Autodesk Inventor part; units mm, degrees
ref_plane "YZ Plane" through (0, 0, 0) normal (1, 0, 0) x (0, 1, 0)
ref_plane "XZ Plane" through (0, 0, 0) normal (0, 1, 0) x (-1, 0, 0)
ref_plane "XY Plane" through (0, 0, 0) normal (0, 0, 1) x (1, 0, 0)
sketch "Sketch1" plane through (0, 0, 0) normal (0, 0, 1) x (1, 0, 0)
  line L0 (-750, 50) -> (750, 50)
  line L1 (750, 50) -> (750, 0)
  line L2 (750, 0) -> (-750, 0)
  line L3 (-750, 0) -> (-750, 50)
  point P0 (0, 0)
  point P1 (0, 0)
  dimension "d0" = 1500
  dimension "d1" = 50
extrude "Plate1" add sketch "Sketch1" along normal blind 3
sketch "Sketch2" plane through (750, 3, 0) normal (0, -1, 0) x (1, 0, 0)
  line L0 (-1500, 0) -> (0, 0)
  line L1 (0, 0) -> (0, 30)
  line L2 (0, 30) -> (-1500, 30)
  line L3 (-1500, 30) -> (-1500, 0)
edge flange "Flange1" height 30 angle 90 thickness 3 bend radius 3 thickness toward (0, -1, 0) relief tear relief width 3 relief depth 1.5 edges at (0, 0, 3) wall of the first edge with corners at (-750, 3, 0) (750, 3, 0) (750, 3, 30) (-750, 3, 30)
bend "Bend1"
corner "Corner1"
sketch "Sketch5" plane through (0, 0, 0) normal (0, 0, -1) x (-1, 0, 0)
  line L0 (750, 50) -> (-750, 50)
  line L1 (497, 50) -> (497, 29)
  line L2 (497, 29) -> (500, 29)
  line L3 (500, 29) -> (500, 50)
  point P0 (0, 0)
  dimension "d17" = 21
  dimension "d18" = 3
  dimension "d19" = 250
extrude "Extrusion1" cut sketch "Sketch5" against normal through all
equation "\"d18\" = Thickness"
equation "\"d2\" = Thickness"
equation "\"d3\" = BendReliefWidth"
equation "\"d4\" = BendReliefDepth"
equation "\"d5\" = MinimumRemnant"
equation "\"d6\" = TransitionRadius"
equation "\"d9\" = BendRadius"
equation "\"d10\" = CornerReliefSize"
equation "\"d11\" = GapSize"
equation "\"d12\" = JacobiRadiusSize"
equation "\"BendRadius\" = Thickness"
equation "\"BendReliefWidth\" = Thickness"
equation "\"BendReliefDepth\" = 0.5 * Thickness"
equation "\"CornerReliefSize\" = 4 * Thickness"
equation "\"MinimumRemnant\" = 2 * Thickness"
equation "\"TransitionRadius\" = BendRadius"
equation "\"JacobiRadiusSize\" = BendRadius"
equation "\"GapSize\" = Thickness"
properties part number "МОО 050 стрингер спина 1"
Geometry check sheet. Reference: the model listing, model coordinates, mm. A direction names the side the tool comes from. Round coordinates to 2 decimals unless told otherwise and drop trailing zeros. Order: outer loops, then holes, each group sorted by start corner. A loop starts at its lowest first (then second) coordinate and runs counter-clockwise, first axis right, second up. Notation, with made-up numbers: M 67.25,43 L 113.25,43 A16 ccw 113.25,69 Z; hole C 28.25,35 d8. An arc over 180 degrees is marked long. Answer in a Markdown table with one row per item. Add a question column.
Item 1: Sectioned sample at C-C, the plane z = 21. Enter the section's corners in (x, y), plus the area to 3 significant figures.
Item 2: Sectioned sample at B-B, the plane x = 128. Enter the section's corners in (y, z).
Item 3: Depth check by flat-ended pin: pin 1 Ø1.5 at (x, z) = (-498, 1) entering from +Y; pin 2 Ø4 at (x, y) = (-305, 14.5) entering from +Z; pin 3 Ø12 at (x, z) = (-206, 24) entering from +Y. Enter the tip coordinate at first touch or a pass-through.
Item 4: Sectioned sample at A-A, the plane y = 41.5. Enter the section's corners in (x, z).
Item 5: Material ranges on L1, parallel to Y at x = 279.5, z = 26.25; L2, parallel to Y at x = 388, z = 1.75, recorded low to high. Write a range as [from, to].
Item 6: Set-up check for faces 1 (the face through (-10, 28, 3)), 2 (the face through (750, 17.5, 2.8)): record each of +Z, -Z, +X, -X, +Y, -Y from which the full face is reachable in a straight line by a thin tool's end or side.
Filled in:
| question | item | result |
|---|---|---|
| 1 | outline | M -750,0 L 750,0 L 750,3 L -750,3 Z |
| 1 | area | 4,500 mm² |
| 2 | outline | M 0,6 A6 ccw 6,0 L 50,0 L 50,3 L 6,3 A3 cw 3,6 L 3,30 L 0,30 Z |
| 3 | pin 1 | stops at y = 29 |
| 3 | pin 2 | stops at z = 3 |
| 3 | pin 3 | stops at y = 3 |
| 4 | outline | M -750,0 L -500,0 L -500,3 L -750,3 Z; M -497,0 L 750,0 L 750,3 L -497,3 Z |
| 5 | L1 | y = [0, 3] |
| 5 | L2 | y = [1.76, 50] |
| 6 | face 1 | +Z, +X, -X, +Y |
| 6 | face 2 | +Z, -Z, +X, +Y, -Y |
